Build history of the part. All positions in model axes, mm. Face numbers are marked on the shaded views. A direction names the side the tool comes from. Round coordinates to 2 decimals unless told otherwise and drop trailing zeros. Write each loop counter-clockwise with the first axis right and the second up, starting at its lowest first coordinate (ties: lowest second). Pieces come first, ordered by that corner, then holes. Notation, with made-up numbers: (4, -27.75) -> (16, -27.75) arc R11 cw to (16, -16.75) -> close; hole circle Ø8 at (56, 1.25). An arc over 180 degrees is marked (long way). Return JSON: item names as keys, results as strings.
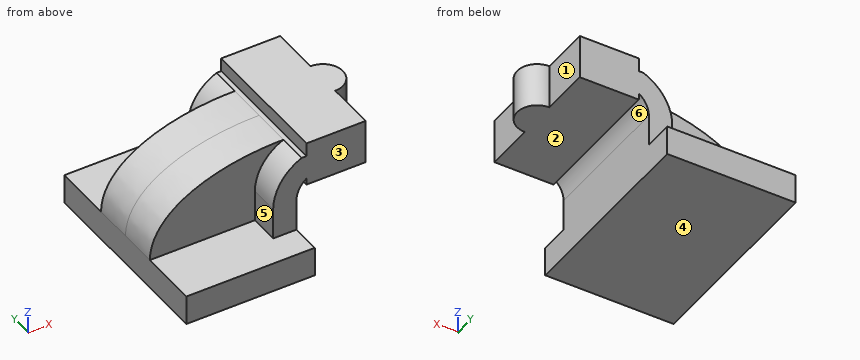
from build123d import *

# Parameters (mm, degrees)
F1_DEPTH = 63.5
F2_DEPTH = 25.4
F0_W     = 37.9670182306
F0_H     = 8.8137983387
F3_DEPTH = 44.45


with BuildPart() as f1:
    # F0 (on Front) → F1 (new body, symmetric)
    with BuildSketch(Plane.XZ):
        Polygon((36.9568020105, 4.2637886968), (-30.6071963282, 4.2637886968), (-30.6071963282, -14.7862113032), (51.9428036718, -14.7862113032), (51.9428036718, 4.2637886968), align=None)
    extrude(amount=F1_DEPTH, both=True)

    # F0 (on Front) → F2 (join, symmetric)
    with BuildSketch(Plane.XZ):
        with BuildLine():
            add(Edge.make_bspline(
                [(-30.6071963282, 4.2637886968), (-29.9851279706, 36.267735064), (10.8517641202, 52.8309457004), (55.3704965091, 52.5999903581)],
                knots=[0, 0, 0, 0, 98.6334226145, 98.6334226145, 98.6334226145, 98.6334226145], degree=3))
            Line((-30.6071963282, 4.2637886968), (36.9568020105, 4.2637886968))
            Line((36.9568020105, 4.2637886968), (36.9568020105, 24.3605504215))
            ThreePointArc((36.9568020105, 24.3605504215), (41.9669062931, 41.2167815618), (55.3704965091, 52.5999903581))
        make_face()
    extrude(amount=F2_DEPTH, both=True)

    # F0 (on Front) → F3 (join, symmetric)
    with BuildSketch(Plane.XZ):
        with BuildLine():
            Line((36.9568020105, 24.3605504215), (36.9568020105, 4.2637886968))
            Line((36.9568020105, 4.2637886968), (51.9428036718, 4.2637886968))
            Line((51.9428036718, 4.2637886968), (51.9428036718, 24.3605504215))
            ThreePointArc((51.9428036718, 24.3605504215), (53.6559903273, 31.5340201394), (58.4257854412, 37.1592073258))
            Line((58.4257854412, 37.1592073258), (58.4257854412, 52.5999903581))
            Line((58.4257854412, 52.5999903581), (55.3704965091, 52.5999903581))
            ThreePointArc((55.3704965091, 52.5999903581), (41.9669062931, 41.2167815618), (36.9568020105, 24.3605504215))
        make_face()
        with BuildLine():
            Line((96.3928036718, 52.5999903581), (58.4257854412, 52.5999903581))
            Line((58.4257854412, 52.5999903581), (58.4257854412, 37.1592073258))
            ThreePointArc((58.4257854412, 37.1592073258), (58.7496754638, 37.3906953095), (59.0792683894, 37.6139886968))
            Line((59.0792683894, 37.6139886968), (96.3928036718, 37.6139886968))
            Line((96.3928036718, 37.6139886968), (96.3928036718, 52.5999903581))
        make_face()
        with BuildLine():
            ThreePointArc((59.0792683894, 37.6139886968), (58.7496754638, 37.3906953095), (58.4257854412, 37.1592073258))
            Line((58.4257854412, 37.1592073258), (58.4257854412, 32.8387886968))
            Line((58.4257854412, 32.8387886968), (96.3928036718, 32.8387886968))
            Line((96.3928036718, 32.8387886968), (96.3928036718, 37.6139886968))
            Line((96.3928036718, 37.6139886968), (59.0792683894, 37.6139886968))
        make_face()
        with Locations((77.4092945565, 57.0068895275)):
            Rectangle(F0_W, F0_H)
    extrude(amount=F3_DEPTH, both=True)

    # F0 (on Front) → F4 (revolve)
    with BuildSketch(Plane.XZ):
        Polygon((96.3928036718, 61.4137886968), (96.3928036718, 52.5999903581), (96.3928036718, 37.6139886968), (96.3928036718, 32.8387886968), (109.2257854412, 32.8387886968), (109.2257854412, 61.4137886968), align=None)
    revolve(axis=Axis((96.3928036718, 0, 49.5138886968), (0, 0, -1)))


solid = f1.part
Q1. Wall check: L1, parallel to Z at x = 95.5, y = -14.5; L2, parallel to Y at x = 48, z = 36.5; L3, parallel to Y at x = 3, z = 30.5. Give the ranges that are in metal, low to high.
Verdict:
{"L1": "z = 32.84 to 61.41", "L2": "y = -44.45 to 44.45", "L3": "y = -25.4 to 25.4"}
Q2. Two-plate mould, pull along X, no slides. Class the marked faces 4, 5 and 6: +X half, -X half, draft (parallel to the pull), parting line (faces both ways), or undercut.
Verdict:
{"face 4": "draft", "face 5": "-X half", "face 6": "undercut"}
Q3. Saw through at A-A on x = 75. List the corners of the cut face in (y, z).
Verdict:
{"outline": "(-44.45, 32.84) -> (44.45, 32.84) -> (44.45, 61.41) -> (-44.45, 61.41) -> close"}
Q4. Pin check, flat tips, straight feed: pin 1 Ø19.5 at (y, z) = (-20, -2) entering from +X; pin 2 Ø14.5 at (y, z) = (-33.5, 49) entering from +X; pin 3 Ø1.3 at (y, z) = (17.5, 35) entering from -X. Stop position of each tip, or through.
Verdict:
{"pin 1": "stops at x = 51.94", "pin 2": "stops at x = 96.39", "pin 3": "stops at x = -14.01"}
Q5. 3-axis set-ups, long thin cutter, end or side, ignore diameter. For the marked faces 1, 2 and 3: which of +Z, -Z, +X, -X, +Y, -Y reach the whole face in a straight line?
Verdict:
{"face 1": "+Z, -Z, +X, +Y", "face 2": "-Z, +X, +Y, -Y", "face 3": "+Z, +X, -X, -Y"}
Q6. Saw through at B-B on z = -2. List the corners of the cut face in (x, y), then the cut area to 3 significant figures.
Verdict:
{"outline": "(-30.61, -63.5) -> (51.94, -63.5) -> (51.94, 63.5) -> (-30.61, 63.5) -> close", "area": "10,500 mm²"}
